Read the model definition and answer for the solid it produces. Units are mm, in the model's axes. Coordinates: 2 decimals unless noted, no trailing zeros. Write each loop counter-clockwise with the first axis right and the second up, starting at its lowest first coordinate (ties: lowest second). Pieces come first, ordered by that corner, then holes. Notation, with made-up numbers: (-21, 18) -> (7, 18) arc R15 cw to (7, 22) -> close; hole circle Ø8 at (31.5, 56). An arc over 180 degrees is marked (long way). Answer as a JSON object with one key per item and string values. Group by question number.
(1) Find section D-D (x = -145.5). Give the vertices of the cut face in (y, z).
(2) Straight lines are drawn through the part: L1, parallel to X at y = -18, z = 19; L2, parallel to Z at x = -155.5, y = -15; L3, parallel to Z at x = -187.5, y = -9. For each, find the intervals that lie inside material, in ascending order.
(3) Find section C-C (y = 3). Give the vertices of the cut face in (x, z), then the cut area to 3 significant figures.
(4) Flat-ended cylindrical pins translate along their axes: P1, Ø4, axis at x = -24, y = -19.5, coming from the +Z side; P2, Ø10, axis at x = -132.842, z = 14.478, coming from the -Y side; P3, Ø9.5, axis at x = 109, y = 15, coming from the +Z side; P4, Ø10, axis at x = -52, z = 63.5, coming from the -Y side. Find the tip coordinate at first contact, or state that the pin passes through.
(5) Find section B-B (y = -17.5). Give the vertices of the cut face in (x, z).
(6) Find section A-A (z = 47). Give the vertices of the cut face in (x, y), then the cut area to 3 significant figures.
from build123d import *

# Parameters (mm, degrees)
SKETCH1_W           = 482.6
SKETCH1_H           = 50.8
BOSS_EXTRUDE1_DEPTH = 69.85
CUT_EXTRUDE2_DEPTH  = 49.022
SKETCH3_W           = 482.6
SKETCH3_H           = 16.002
CUT_EXTRUDE3_DEPTH  = 31.75
SKETCH4_W           = 482.6
SKETCH4_H           = 15.748
CUT_EXTRUDE4_DEPTH  = 12.7
SHELL2_START        = -23.622
SHELL2_OUTLINE_W    = 479.044
SHELL2_OUTLINE_H    = 14.224
SHELL2_DEPTH        = 47.244
SKETCH5_W           = 1.778
SKETCH5_H           = 17.272
BOSS_EXTRUDE2_DEPTH = 44.45
FILLET1_R           = 2.54
SKETCH6_R           = 3.81
CUT_EXTRUDE5_DEPTH  = 44.45


# Read off the part's stored shape, not the designer's step: Shell2
with BuildPart() as part:
    # Sketch1 → Boss-Extrude1 (new body)
    with BuildSketch(Plane.XY):
        Rectangle(SKETCH1_W, SKETCH1_H)
    extrude(amount=BOSS_EXTRUDE1_DEPTH)

    # Sketch2 → Cut-Extrude2 (cut)
    with BuildSketch(Plane(origin=(0, 25.4, 0), x_dir=(1, 0, 0), z_dir=(0, 1, 0))):
        Polygon((241.3, -16.002), (-241.3, -16.002), (-241.3, -34.925), (-241.3, -53.848), (241.3, -53.848), align=None)
    extrude(amount=-CUT_EXTRUDE2_DEPTH, mode=Mode.SUBTRACT)

    # Sketch3 → Cut-Extrude3 (cut)
    with BuildSketch(Plane(origin=(0, 25.4, 0), x_dir=(1, 0, 0), z_dir=(0, 1, 0))):
        with Locations((0, -61.849)):
            Rectangle(SKETCH3_W, SKETCH3_H)
    extrude(amount=-CUT_EXTRUDE3_DEPTH, mode=Mode.SUBTRACT)

    # Sketch4 → Cut-Extrude4 (cut)
    with BuildSketch(Plane.XY.offset(69.85)):
        with Locations((0, -17.526)):
            Rectangle(SKETCH4_W, SKETCH4_H)
    extrude(amount=-CUT_EXTRUDE4_DEPTH, mode=Mode.SUBTRACT)

    # Shell2 outline → Shell2 (cut)
    with BuildSketch(Plane(origin=(0, 0, 0), x_dir=(1, 0, 0), z_dir=(0, 1, 0)).offset(SHELL2_START)):
        with Locations((0, -8.89)):
            Rectangle(SHELL2_OUTLINE_W, SHELL2_OUTLINE_H)
    extrude(amount=SHELL2_DEPTH, mode=Mode.SUBTRACT)

    # Sketch5 → Boss-Extrude2 (add)
    with BuildSketch(Plane(origin=(0, 0, 53.848), x_dir=(-1, 0, 0), z_dir=(0, 0, -1))):
        with Locations((240.411, -14.986)):
            Rectangle(SKETCH5_W, SKETCH5_H)
        with Locations((-240.411, -14.986)):
            Rectangle(SKETCH5_W, SKETCH5_H)
    extrude(amount=BOSS_EXTRUDE2_DEPTH)

    # Fillet1
    fillet1_edges = [part.edges().sort_by_distance(p)[0] for p in [
        (0, -25.4, 0),
        (0, -25.4, 57.15),
        (0, 25.4, 0),
        (0, -6.35, 53.848),
    ]]
    fillet(fillet1_edges, radius=FILLET1_R)

    # Sketch6 → Cut-Extrude5 (cut)
    with BuildSketch(Plane(origin=(0, -23.622, 0), x_dir=(1, 0, 0), z_dir=(0, 1, 0))):
        with Locations(Location((-132.842, -14.478, 0), (0, 0, 270))):
            Circle(SKETCH6_R)
        with Locations(Location((132.842, -14.478, 0), (0, 0, 270))):
            Circle(SKETCH6_R)
    extrude(amount=-CUT_EXTRUDE5_DEPTH, mode=Mode.SUBTRACT)


solid = part.part
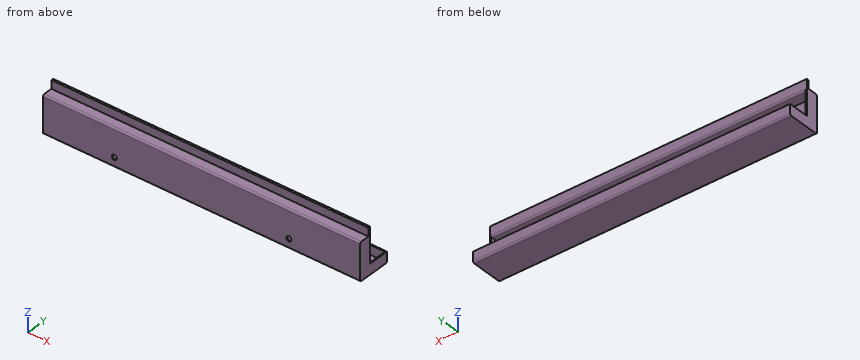
Results below:
{
 "1": {"outline": "(-25.4, 2.54) arc R2.54 ccw to (-22.86, 0) -> (22.86, 0) arc R2.54 ccw to (25.4, 2.54) -> (25.4, 16) -> (23.62, 16) -> (23.62, 1.78) -> (-23.62, 1.78) -> (-23.62, 53.85) -> (-8.89, 53.85) arc R2.54 ccw to (-6.35, 56.39) -> (-6.35, 69.85) -> (-9.65, 69.85) -> (-9.65, 57.15) -> (-22.86, 57.15) arc R2.54 ccw to (-25.4, 54.61) -> close"},
 "2": {"L1": "x = -241.3 to -239.52, 239.52 to 241.3", "L2": "z = 0 to 1.78, 53.85 to 57.15", "L3": "z = 0 to 1.78, 53.85 to 69.85"},
 "3": {"outline": "(-241.3, 0) -> (241.3, 0) -> (241.3, 16) -> (239.52, 16) -> (239.52, 1.78) -> (-239.52, 1.78) -> (-239.52, 16) -> (-241.3, 16) -> close", "area": "909 mm2"},
 "4": {"P1": "stops at z = 57.15", "P2": "stops at y = -25.4", "P3": "stops at z = 1.78", "P4": "stops at y = -9.65"},
 "5": {"outline": "(-241.3, 0) -> (241.3, 0) -> (241.3, 57.15) -> (-241.3, 57.15) -> close; hole (-239.52, 1.78) -> (239.52, 1.78) -> (239.52, 53.85) -> (-239.52, 53.85) -> close"},
 "6": {"outline": "(-241.3, -25.4) -> (241.3, -25.4) -> (241.3, -6.35) -> (239.52, -6.35) -> (239.52, -23.62) -> (-239.52, -23.62) -> (-239.52, -6.35) -> (-241.3, -6.35) -> close", "area": "919 mm2"}
}
